The model under review builds one solid part; all positions refer to its coordinate system, in mm. Face numbers are marked on the shaded views. A direction names the side the tool comes from. Coordinates: 2 decimals unless noted, no trailing zeros. Order: outer loops, then holes, each group sorted by start corner. A loop starts at its lowest first (then second) coordinate and runs counter-clockwise, first axis right, second up. Notation, with made-up numbers: (-24.5, 83.25) - (27.5, 83.25) arc R19 ccw to (27.5, 105.25) - close; hole circle Ø11 at (64, 63). An arc over 180 degrees is marked (long way). Answer in a Markdown table with one row per item.
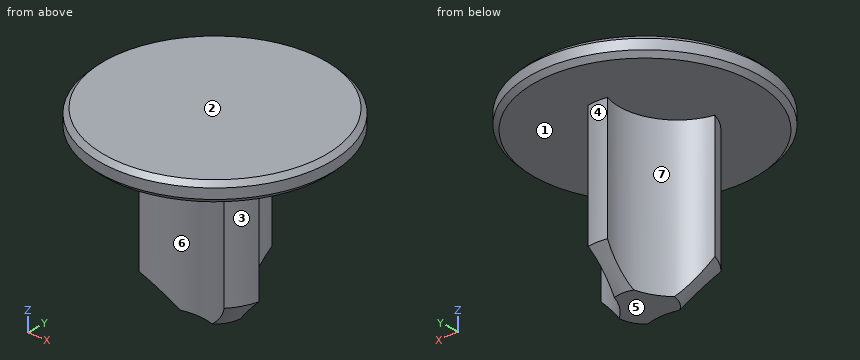
```python
from build123d import *

# Parameters (mm, degrees)
F0_W     = 9.525
F0_H     = 25.4
F2_SIZE  = 0.762
F3_R     = 9.525
F4_DEPTH = 25.4
F5_SIZE  = 5.08


with BuildPart() as f1:
    # F0 (on Front) → F1 (revolve)
    with BuildSketch(Plane.XZ):
        with Locations((-4.7625, -12.7)):
            Rectangle(F0_W, F0_H)
        Polygon((-9.525, 0), (0, 0), (0, 3.175), (-19.05, 3.175), (-19.05, 0), align=None)
    revolve(axis=Axis((0, 0, -12.7), (0, 0, -1)))

    # F2
    f2_edges = [f1.edges().sort_by_distance(p)[0] for p in [
        (19.05, 0, 0),
        (19.05, 0, 3.175),
    ]]
    chamfer(f2_edges, length=F2_SIZE)

    # F3 (on face) → F4 (cut, through all)
    with BuildSketch(Plane(origin=(0, 0, -25.4), x_dir=(1, 0, 0), z_dir=(0, 0, -1))):
        with Locations((0, 12.7)):
            Circle(F3_R)
        with Locations((-10.9985226281, -6.35)):
            Circle(F3_R)
        with Locations((10.4095544736, -7.2753814788)):
            Circle(F3_R)
    extrude(amount=-F4_DEPTH, mode=Mode.SUBTRACT)

    # F5
    f5_edges = [f1.edges().sort_by_distance(p)[0] for p in [
        (-8.248892, -4.7625, -25.4),
        (-0.411342, 9.516114, -25.4),
        (8.446867, -4.401825, -25.4),
    ]]
    chamfer(f5_edges, length=F5_SIZE)


solid = f1.part
```
Item 1: We need section A-A, the plane x = 0. Write out the cut boundary in (y, z) (3 decimals), then the cut area to 3 significant figures.
Check values:
| item | result |
|---|---|
| outline | (-19.05, 0.762) - (-18.288, 0) - (-3.175, 0) - (-3.175, -25.4) - (4.445, -25.4) - (9.525, -20.32) - (9.525, 0) - (18.288, 0) - (19.05, 0.762) - (19.05, 2.413) - (18.288, 3.175) - (-18.288, 3.175) - (-19.05, 2.413) - close |
| area | 429 mm^2 |
Item 2: Mouldability with a two-part tool opening along Y and no side actions: class the marked faces 5, 6 and 7 as +Y half, -Y half, draft (parallel to the pull), parting line (faces both ways), or undercut.
Check values:
| item | result |
|---|---|
| face 5 | draft |
| face 6 | -Y half |
| face 7 | undercut |
Item 3: Tool access review of the marked faces 1, 2, 3 and 4: name each direction out of +Z, -Z, +X, -X, +Y, -Y from which nothing blocks a thin tool from reaching the whole face with its end or side.
Check values:
| item | result |
|---|---|
| face 1 | -Z |
| face 2 | +Z, +X, -X, +Y, -Y |
| face 3 | -Z, +X, -Y |
| face 4 | -Z, +Y |
Item 4: Clearance check with flat-ended pins moving along their axes: pin 1 Ø10 at (x, y) = (11, 4) entering from -Z; pin 2 Ø8 at (y, z) = (2.5, -15.5) entering from +X; pin 3 Ø10 at (y, z) = (5, -15.5) entering from -X. State where each tip first meets the part, or that it passes through.
Check values:
| item | result |
|---|---|
| pin 1 | z = 0 |
| pin 2 | x = 6.71 |
| pin 3 | x = -3.9 |
Item 5: To check wall thickness, follow line 1 (Z direction, x = -16.5, y = 1) (3 decimals); line 2 (Y direction, x = 8.5, z = -0.75); line 3 (X direction, y = 8.5, z = -18.5). State the ranges of each line that lie inside material, in increasing order. Write a range as from..to.
Check values:
| item | result |
|---|---|
| line 1 | 0..3.175 |
| line 2 | -4.3..-2.06 |
| line 3 | -1.72..0.96 |
